from build123d import *

# Parameters (mm, degrees)
SKETCH_2_W          = 21.686450318
SKETCH_2_H          = 18.975644028
EXTRUDE_1_DEPTH     = 80
SKETCH_3_W          = 4.325856272
SKETCH_3_H          = 3.850004403
SKETCH_3_W_2        = 5.584754458
SKETCH_3_W_3        = 3.96682231
SKETCH_3_H_2        = 3.692656783
SKETCH_3_W_4        = 4.705718876
SKETCH_3_H_3        = 4.627145628
SKETCH_3_W_5        = 4.481794252
SKETCH_3_H_4        = 4.742838382
SKETCH_3_W_6        = 4.224308281
SKETCH_3_H_5        = 4.189521493
SKETCH_3_W_7        = 4.472125562
SKETCH_3_H_6        = 4.472586404
SKETCH_3_W_8        = 5.542155091
SKETCH_3_H_7        = 4.001347562
CUT_EXTRUDE_1_DEPTH = 2
SKETCH_4_W          = 3.008522681
SKETCH_4_H          = 2.673197864
SKETCH_4_W_2        = 5.706300448
SKETCH_4_H_2        = 3.399675438
SKETCH_4_W_3        = 6.296507583
SKETCH_4_H_3        = 3.509528199
SKETCH_4_W_4        = 4.633699799
SKETCH_4_H_4        = 4.622885298
SKETCH_4_W_5        = 3.431694386
SKETCH_4_H_5        = 3.11922744
SKETCH_4_W_6        = 7.114178537
SKETCH_4_H_6        = 3.614354853
SKETCH_4_W_7        = 5.071310287
SKETCH_4_H_7        = 3.04134768
CUT_EXTRUDE_2_DEPTH = 2


with BuildPart() as part:
    # Эскиз2 → Бобышка-Вытянуть1 (new body)
    with BuildSketch(Plane(origin=(0, 0, 0), x_dir=(1, 0, 0), z_dir=(0, 1, 0))):
        with Locations((-10.843225159, 9.487822014)):
            Rectangle(SKETCH_2_W, SKETCH_2_H)
    extrude(amount=EXTRUDE_1_DEPTH)

    # Эскиз3 → Вырез-Вытянуть1 (cut)
    with BuildSketch(Plane.XY):
        with Locations((-16.546390401, 73.000252652)):
            Rectangle(SKETCH_3_W, SKETCH_3_H)
        with Locations((-6.133816144, 73.000252652)):
            Rectangle(SKETCH_3_W_2, SKETCH_3_H)
        with Locations((-15.486029562, 64.011252425)):
            Rectangle(SKETCH_3_W_3, SKETCH_3_H_2)
        with Locations((-6.573333935, 63.544008002)):
            Rectangle(SKETCH_3_W_4, SKETCH_3_H_3)
        with Locations((-13.245132436, 52.626011155)):
            Rectangle(SKETCH_3_W_5, SKETCH_3_H_4)
        with Locations((-15.357286577, 42.478535232)):
            Rectangle(SKETCH_3_W_6, SKETCH_3_H_5)
        with Locations((-5.577501696, 41.464970569)):
            Rectangle(SKETCH_3_W_7, SKETCH_3_H_6)
        with Locations((-13.775312856, 32.542849067)):
            Rectangle(SKETCH_3_W_8, SKETCH_3_H_7)
    extrude(amount=-CUT_EXTRUDE_1_DEPTH, mode=Mode.SUBTRACT)

    # Эскиз4 → Вырез-Вытянуть2 (cut)
    with BuildSketch(Plane(origin=(0, 0, 0), x_dir=(0, 0, -1), z_dir=(1, 0, 0))):
        with Locations((4.831613066, 72.817657134)):
            Rectangle(SKETCH_4_W, SKETCH_4_H)
        with Locations((14.543739986, 72.454418347)):
            Rectangle(SKETCH_4_W_2, SKETCH_4_H_2)
        with Locations((8.54233597, 65.380205413)):
            Rectangle(SKETCH_4_W_3, SKETCH_4_H_3)
        with Locations((5.034477327, 55.62228831)):
            Rectangle(SKETCH_4_W_4, SKETCH_4_H_4)
        with Locations((15.046052856, 54.870459381)):
            Rectangle(SKETCH_4_W_5, SKETCH_4_H_5)
        with Locations((6.884440994, 46.683688672)):
            Rectangle(SKETCH_4_W_6, SKETCH_4_H_6)
        with Locations((14.226244905, 39.396398085)):
            Rectangle(SKETCH_4_W_7, SKETCH_4_H_7)
    extrude(amount=-CUT_EXTRUDE_2_DEPTH, mode=Mode.SUBTRACT)


solid = part.part
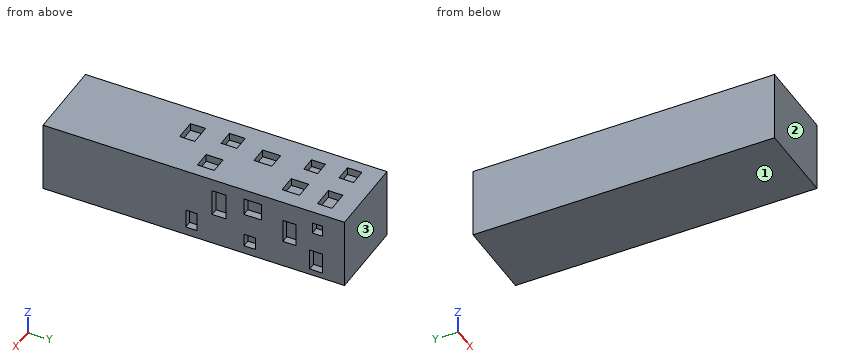
Geometry: final body of the model. Coordinates: model frame, mm. Face numbers are marked on the shaded views. Round coordinates to 2 decimals unless told otherwise and drop trailing zeros. Order: outer loops, then holes, each group sorted by start corner. A loop starts at its lowest first (then second) coordinate and runs counter-clockwise, first axis right, second up. Notation, with made-up numbers: (87, -15) -> (135, -15) arc R24 ccw to (135, 24) -> close; hole circle Ø10 at (11.25, -33). An arc over 180 degrees is marked (long way). Put each result on its own line as item: value. Start each with the question number.
Q1. Pull-direction query (Y, two-part tool) for the marked faces 1, 2 and 3; classes: +Y half, -Y half, draft (parallel to the pull), parting line (faces both ways), or undercut.
Q2. Line query: probe 1 along X at (y, z) = (53.5, -5.25); probe 2 along Z at (x, y) = (-5.75, 64.5). Output: solid intervals per line, ascending.
Q3. Section B-B on y = 64.5. Return the cut outline in (x, z), and give its area (3 significant figures).
Q4. First-contact query: pin 1 (1.8 mm diameter, centred on y = 46.5, z = -8.5, fed in from +X). Flat tip, straight axial feed; report the tip coordinate or a pass-through.
Q5. Section A-A on x = -1.25. Give the number of separate pieces and of enclosed holes in the cut face, and give its area (3 significant figures).
Ans:
1. face 1: draft
1. face 2: -Y half
1. face 3: +Y half
2. probe 1: x = -21.69 to -2
2. probe 2: z = -18.98 to -2
3. outline: (-21.69, -18.98) -> (0, -18.98) -> (0, -11.69) -> (-2, -11.69) -> (-2, -5.39) -> (0, -5.39) -> (0, 0) -> (-4.22, 0) -> (-4.22, -2) -> (-8.93, -2) -> (-8.93, 0) -> (-13.5, 0) -> (-13.5, -2) -> (-17.47, -2) -> (-17.47, 0) -> (-21.69, 0) -> close
3. area: 382 mm2
4. pin 1: stops at x = -2
5. separate pieces: 1
5. enclosed holes: 7
5. area: 1,400 mm2
